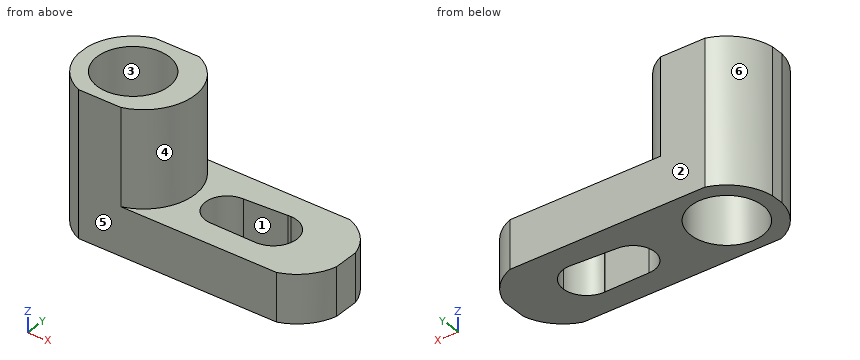
```python
from build123d import *

# Parameters (mm, degrees)
F0_W     = 69.85
F0_H     = 38.1
F1_DEPTH = 25.4
F3_DEPTH = 38.101
F5_DEPTH = 25.4
F6_R     = 9.503883
F7_DEPTH = 38.101
F9_DEPTH = 12.701


with BuildPart() as f1:
    # F0 (on Front) → F1 (new body)
    with BuildSketch(Plane.XZ):
        with Locations((-7.206795, 19.05)):
            Rectangle(F0_W, F0_H)
    extrude(amount=F1_DEPTH)

    # F2 (on face) → F3 (cut, through all)
    with BuildSketch(Plane.XY.offset(38.1)):
        with BuildLine():
            ThreePointArc((-42.131795, -11.242362), (-39.065027, -4.218313), (-32.665953, 0))
            Line((-32.665953, 0), (-42.131795, 0))
            Line((-42.131795, 0), (-42.131795, -11.242362))
        make_face()
        with BuildLine():
            ThreePointArc((-33.817176, -25.4), (-39.447694, -21.112905), (-42.131795, -14.564811))
            Line((-42.131795, -14.564811), (-42.131795, -25.4))
            Line((-42.131795, -25.4), (-33.817176, -25.4))
        make_face()
        with BuildLine():
            Line((27.718205, -25.4), (27.718205, -15.992137))
            ThreePointArc((27.718205, -15.992137), (24.495171, -21.836901), (18.851276, -25.4))
            Line((18.851276, -25.4), (27.718205, -25.4))
        make_face()
        with BuildLine():
            Line((27.718205, 0), (19.139083, 0))
            ThreePointArc((19.139083, 0), (24.598614, -3.577897), (27.718205, -9.311655))
            Line((27.718205, -9.311655), (27.718205, 0))
        make_face()
    extrude(amount=-F3_DEPTH, mode=Mode.SUBTRACT)

    # F4 (on face) → F5 (cut)
    with BuildSketch(Plane.XY.offset(38.1)):
        with BuildLine():
            ThreePointArc((-20.865917, 0), (-12.835523, -13.304651), (-22.592751, -25.4))
            Line((-22.592751, -25.4), (18.851276, -25.4))
            ThreePointArc((18.851276, -25.4), (24.495171, -21.836901), (27.718205, -15.992137))
            Line((27.718205, -15.992137), (27.718205, -9.311655))
            ThreePointArc((27.718205, -9.311655), (24.598614, -3.577897), (19.139083, 0))
            Line((19.139083, 0), (-20.865917, 0))
        make_face()
    extrude(amount=-F5_DEPTH, mode=Mode.SUBTRACT)

    # F6 (on face) → F7 (cut, through all)
    with BuildSketch(Plane.XY.offset(38.1)):
        with Locations((-28.749728, -12.903587)):
            Circle(F6_R)
    extrude(amount=-F7_DEPTH, mode=Mode.SUBTRACT)

    # F8 (on face) → F9 (cut, through all)
    with BuildSketch(Plane.XY.offset(12.7)):
        with BuildLine():
            ThreePointArc((-3.597571, -18.851277), (0.472617, -17.16535), (2.158544, -13.095162))
            ThreePointArc((2.158544, -13.095162), (0.472617, -9.024974), (-3.597571, -7.339047))
            ThreePointArc((-3.597571, -7.339047), (-9.353686, -13.095162), (-3.597571, -18.851277))
        make_face()
        with BuildLine():
            ThreePointArc((-3.597571, -7.339047), (0.472617, -9.024974), (2.158544, -13.095162))
            ThreePointArc((2.158544, -13.095162), (0.472617, -17.16535), (-3.597571, -18.851277))
            Line((-3.597571, -18.851277), (8.330685, -19.004828))
            ThreePointArc((8.330685, -19.004828), (2.29775, -13.102009), (7.742962, -6.653036))
            Line((7.742962, -6.653036), (-3.597571, -7.339047))
        make_face()
        with BuildLine():
            Line((8.49027, -6.60783), (7.742962, -6.653036))
            ThreePointArc((7.742962, -6.653036), (2.29775, -13.102009), (8.330685, -19.004828))
            Line((8.330685, -19.004828), (8.49027, -19.006882))
            ThreePointArc((8.49027, -19.006882), (12.873997, -17.191083), (14.689796, -12.807356))
            ThreePointArc((14.689796, -12.807356), (12.873997, -8.423629), (8.49027, -6.60783))
        make_face()
        with BuildLine():
            ThreePointArc((8.49027, -6.60783), (8.115933, -6.619142), (7.742962, -6.653036))
            Line((7.742962, -6.653036), (8.49027, -6.60783))
        make_face()
        with BuildLine():
            Line((8.49027, -19.006882), (8.330685, -19.004828))
            ThreePointArc((8.330685, -19.004828), (8.410471, -19.006368), (8.49027, -19.006882))
        make_face()
    extrude(amount=-F9_DEPTH, mode=Mode.SUBTRACT)


solid = f1.part
```
Can you work these out from the model? Positions are in its coordinate system, mm. Face numbers are marked on the shaded views. A direction names the side the tool comes from. Coordinates: 2 decimals unless noted, no trailing zeros. Loops run counter-clockwise (first coordinate to the right, second up) from the corner with the lowest first, then second, coordinate; pieces in that order, holes last.
1) For pin 1 (6 mm diameter, centred on y = -19.5, z = 9.5, fed in from -X); pin 2 (2 mm diameter, centred on y = -20.5, z = 16.5, fed in from -X); pin 3 (4 mm diameter, centred on y = -18.5, z = 19, fed in from +X), each with a flat end and sliding along its axis, tell me the tip position at first contact or that it passes through.
2) Imagine slicing it at B-B on z = 28.5. List the corners of the cut face in (x, y) for me.
3) Imagine slicing it at C-C on y = -21.5. List the corners of the cut face in (x, z) for me, plus the area to 3 significant figures.
4) Imagine slicing it at D-D on x = 13.5. List the corners of the cut face in (y, z) for me, plus the area to 3 significant figures.
5) Imagine slicing it at A-A on x = -2. List the corners of the cut face in (y, z) for me, plus the area to 3 significant figures.
6) I need wall thicknesses on probe 1 along X at (y, z) = (-13, 9); probe 2 along X at (y, z) = (-12.75, 4); probe 3 along Y at (x, z) = (-4, 11). Which ranges of each line are inside material? Lowest first, please.
7) Which directions (+Z, -Z, +X, -X, +Y, -Y) give clear straight access to the entire face, cutting with the end or side of a thin tool? Please do the marked faces 1 and 2.
8) Thinking about a two-plate mould opening in X: for the marked faces 3, 4, 5 and 6, which applies, pulls with the +X half, pulls with the -X half, needs draft (parallel to the pull), parting line crosses it, or undercut?
Completed:
1. pin 1: stops at x = -41.75
1. pin 2: stops at x = -40.51
1. pin 3: stops at x = -13.44
2. outline: (-42.13, -14.56) arc R13.48 ccw to (-33.82, -25.4) - (-22.59, -25.4) arc R13.55 ccw to (-20.87, 0) - (-32.67, 0) arc R13.48 ccw to (-42.13, -11.24) - close; hole circle Ø19.01 at (-28.75, -12.9)
3. outline: (-39.14, 0) - (-32.8, 0) - (-32.8, 38.1) - (-39.14, 38.1) - close; (-24.7, 0) - (24.8, 0) - (24.8, 12.7) - (-16.33, 12.7) - (-16.33, 38.1) - (-24.7, 38.1) - close
3. area: 1,080 mm2
4. outline: (-25.4, 0) - (-16.46, 0) - (-16.46, 12.7) - (-25.4, 12.7) - close; (-9.16, 0) - (0, 0) - (0, 12.7) - (-9.16, 12.7) - close
4. area: 230 mm2
5. outline: (-25.4, 0) - (-18.87, 0) - (-18.87, 12.7) - (-25.4, 12.7) - close; (-7.24, 0) - (0, 0) - (0, 12.7) - (-7.24, 12.7) - close
5. area: 175 mm2
6. probe 1: x = -42.13 to -38.25, -19.25 to -9.35, 14.69 to 27.72
6. probe 2: x = -42.13 to -38.25, -19.25 to -9.34, 14.69 to 27.72
6. probe 3: y = -25.4 to -18.84, -7.35 to 0
7. face 1: +Z, -Z
7. face 2: +Z, -Z, +X, -X, +Y
8. face 3: undercut
8. face 4: pulls with the +X half
8. face 5: needs draft
8. face 6: pulls with the -X half
